Here's how the part is built. I have some questions about the finished solid (model axes, mm). A direction names the side the tool comes from. Round coordinates to 2 decimals unless told otherwise and drop trailing zeros. Order: outer loops, then holes, each group sorted by start corner. A loop starts at its lowest first (then second) coordinate and runs counter-clockwise, first axis right, second up. Notation, with made-up numbers: (83.5, -10) - (119.5, -10) arc R19 cw to (119.5, 1) - close; hole circle Ø11 at (-17.75, 23.5). An arc over 180 degrees is marked (long way). Answer as a JSON object with one key per item and string values.
```python
from build123d import *

# Parameters (mm, degrees)
F1_DEPTH = 2
F2_R     = 5.99999
F3_R     = 1
F4_R     = 10.5
F5_DEPTH = 4.001
F7_DEPTH = 1.4


# Not quite as in the source:
# - a fillet or chamfer is up to 0.001 mm smaller than in the source, because OpenCascade refuses the exact size


with BuildPart() as f1:
    # F0 (on Top) → F1 (new body, symmetric)
    with BuildSketch(Plane.XY):
        with BuildLine():
            ThreePointArc((-6, 11.5325625947), (-6.7453687816, -11.1130553854), (13, 0))
            ThreePointArc((13, 0), (11.1130553854, 6.7453687816), (6, 11.5325625947))
            Line((6, 11.5325625947), (-6, 11.5325625947))
        make_face()
        with BuildLine():
            Line((-6, 11.5325625947), (6, 11.5325625947))
            ThreePointArc((6, 11.5325625947), (3.5026447844, 12.5192443667), (0.8558504936, 12.9717970973))
            ThreePointArc((0.8558504936, 12.9717970973), (0, 12.8325625947), (-0.8558504936, 12.9717970973))
            ThreePointArc((-0.8558504936, 12.9717970973), (-3.5026447844, 12.5192443667), (-6, 11.5325625947))
        make_face()
        with BuildLine():
            ThreePointArc((0.8558504936, 12.9717970973), (3.5026447844, 12.5192443667), (6, 11.5325625947))
            Line((6, 11.5325625947), (6, 21.5325625947))
            Line((6, 21.5325625947), (-6, 21.5325625947))
            Line((-6, 21.5325625947), (-6, 11.5325625947))
            ThreePointArc((-6, 11.5325625947), (-3.5026447844, 12.5192443667), (-0.8558504936, 12.9717970973))
            ThreePointArc((-0.8558504936, 12.9717970973), (-1.5778472149, 17.7235436914), (2.7, 15.5325625947))
            ThreePointArc((2.7, 15.5325625947), (2.1909810967, 13.9547153797), (0.8558504936, 12.9717970973))
        make_face()
    extrude(amount=F1_DEPTH, both=True)

    # F2 (radius 6 in the source; OpenCascade refuses exactly that, so slightly less here)
    f2_edges = [f1.edges().sort_by_distance(p)[0] for p in [
        (-6, 21.532563, 0),
        (6, 21.532563, 0),
        (6, 11.532563, 0),
        (-6, 11.532563, 0),
    ]]
    fillet(f2_edges, radius=F2_R)

    # F3
    f3_edges = [f1.edges().sort_by_distance(p)[0] for p in [
        (0.85585, 18.093328, 2),
        (0.85585, 18.093328, -2),
    ]]
    fillet(f3_edges, radius=F3_R)

    # F4 (on face) → F5 (cut, through all)
    with BuildSketch(Plane.XY.offset(2)):
        with Locations((0, -3.5)):
            Circle(F4_R)
    extrude(amount=-F5_DEPTH, mode=Mode.SUBTRACT)

    # F6 (on Top) → F7 (cut, symmetric)
    with BuildSketch(Plane.XY):
        with BuildLine():
            ThreePointArc((11, -3.6981110043), (11.452751307, -1.8736361707), (11.605, 0))
            ThreePointArc((11.605, 0), (-1.8736361707, 11.452751307), (-11, -3.6981110043))
            Line((-11, -3.6981110043), (11, -3.6981110043))
        make_face()
        with BuildLine():
            Line((11, -3.6981110043), (-11, -3.6981110043))
            ThreePointArc((-11, -3.6981110043), (0, -11.605), (11, -3.6981110043))
        make_face()
        with BuildLine():
            ThreePointArc((11, -3.6981110043), (0, -11.605), (-11, -3.6981110043))
            Line((-11, -3.6981110043), (-11, -14.1476519146))
            Line((-11, -14.1476519146), (11, -14.1476519146))
            Line((11, -14.1476519146), (11, -3.6981110043))
        make_face()
    extrude(amount=F7_DEPTH, both=True, mode=Mode.SUBTRACT)


solid = f1.part
```
1. If I drill on L1, parallel to Z at x = -10, y = 5; L2, parallel to X at y = 6, z = 1.15; L3, parallel to X at y = 6.5, z = 0.8, over which ranges is the centre line in solid material (lowest first)? Write a range as [from, to].
Responses:
{"L1": "[-2, -1.4], [1.4, 2]", "L2": "[-11.53, -9.93], [9.93, 11.53]", "L3": "[-11.26, -9.61], [9.61, 11.26]"}
2. Imagine slicing it at C-C (y = 6). List the corners of the cut face in (x, z) for me.
Responses:
{"outline": "(-11.53, -2) - (-4.47, -2) - (-4.47, -1.4) - (-9.93, -1.4) - (-9.93, 1.4) - (-4.47, 1.4) - (-4.47, 2) - (-11.53, 2) - close; (4.47, -2) - (11.53, -2) - (11.53, 2) - (4.47, 2) - (4.47, 1.4) - (9.93, 1.4) - (9.93, -1.4) - (4.47, -1.4) - close"}
3. For P1, Ø2, axis at y = -6, z = -0.5, coming from the +X side; P2, Ø1, axis at y = 16.5, z = -1.5, coming from the -X side; P3, Ø1, axis at y = 11.5, z = -0.5, coming from the -X side, each with a flat end and sliding along its axis, tell me the tip position at first contact or that it passes through.
Responses:
{"P1": "x = 12", "P2": "x = -5.98", "P3": "x = -7.3"}
4. Imagine slicing it at B-B (x = 9). List the corners of the cut face in (y, z) for me.
Responses:
{"outline": "(-9.38, -2) - (-8.91, -2) - (-8.91, -1.4) - (-9.38, -1.4) - close; (-9.38, 1.4) - (-8.91, 1.4) - (-8.91, 2) - (-9.38, 2) - close; (1.91, -2) - (9.38, -2) - (9.38, 2) - (1.91, 2) - (1.91, 1.4) - (7.33, 1.4) - (7.33, -1.4) - (1.91, -1.4) - close"}
5. Thinking about a two-plate mould opening in X: for faces 4 (the face through (4.2, 19.82, -0.03)), 5 (the face through (0.332, 6.995, -1.696)), 6 (the face through (-6.6, 12.12, -0.03)), which applies, pulls with the +X half, pulls with the -X half, needs draft (parallel to the pull), parting line crosses it, or undercut?
Responses:
{"face 4": "pulls with the +X half", "face 5": "undercut", "face 6": "pulls with the -X half"}
6. For faces 1 (the face through (11, -5, 0)), 2 (the face through (0.3, 11.6, 0)), 3 (the face through (-6, 15, 0)), which set-ups out of +Z, -Z, +X, -X, +Y, -Y let a thin tool reach every point of the face, with its end or its side?
Responses:
{"face 1": "-Y", "face 2": "none", "face 3": "+Z, -Z, -X, +Y"}
7. Imagine slicing it at D-D (y = 11). List the corners of the cut face in (x, z) for me, plus the area to 3 significant figures.
Responses:
{"outline": "(-7.3, -2) - (7.3, -2) - (7.3, 2) - (-7.3, 2) - close; hole (-3.7, -1.4) - (3.7, -1.4) - (3.7, 1.4) - (-3.7, 1.4) - close", "area": "37.7 mm2"}
